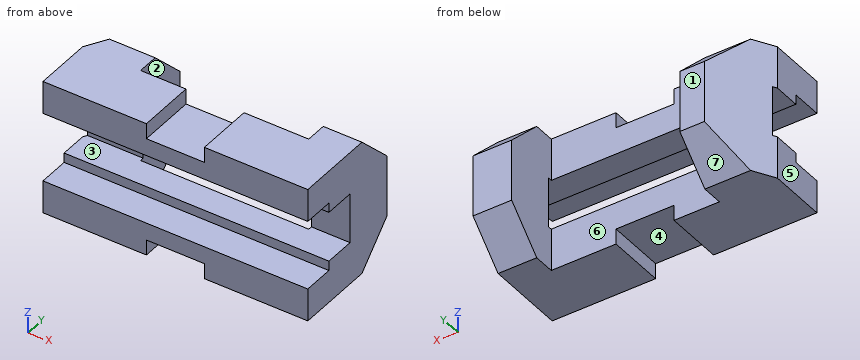
Autodesk Inventor part; units mm, degrees
ref_plane "YZ Plane" through (0, 0, 0) normal (1, 0, 0) x (0, 1, 0)
ref_plane "XZ Plane" through (0, 0, 0) normal (0, 1, 0) x (-1, 0, 0)
ref_plane "XY Plane" through (0, 0, 0) normal (0, 0, 1) x (1, 0, 0)
sketch "草圖1" plane through (0, 0, 0) normal (1, 0, 0) x (0, 1, 0)
  line L0 (-32, 35) -> (9, 35)
  line L1 (9, 35) -> (28, 16)
  line L2 (28, 16) -> (28, 0)
  line L3 (-32, 35) -> (-32, 18)
  line L4 (-32, 18) -> (-16, 18)
  line L5 (-16, 18) -> (-16, 13)
  line L6 (-16, 13) -> (0, 13)
  line L7 (0, 13) -> (0, 6.0328)
  line L8 (28, 0) -> (52.708, 0)
  line L9 (-32, -35) -> (9, -35)
  line L10 (9, -35) -> (28, -16)
  line L11 (28, -16) -> (28, 0)
  line L12 (-32, -35) -> (-32, -18)
  line L13 (-32, -18) -> (-16, -18)
  line L14 (-16, -18) -> (-16, -13)
  line L15 (-16, -13) -> (0, -13)
  line L16 (0, -13) -> (0, 6.0328)
  point P0 (0, 0)
  dimension "d0" = 19
  dimension "d1" = 70
  dimension "d2" = 26
  dimension "d3" = 36
  dimension "d4" = 32
  dimension "d5" = 60
  dimension "d6" = 16
  dimension "d7" = 0
  dimension "d8" = 19
extrude "擠出1" add sketch "草圖1" against normal blind 137
sketch "草圖2" plane through (0, -32, 35) normal (0, 0, 1) x (1, 0, 0)
  line L0 (-137, 0) -> (-137, 41)
  line L1 (-137, 30) -> (-119.6795, 60)
  line L2 (0, 60) -> (-137, 60)
  line L3 (-137, 60) -> (-137, 30)
  line L4 (-119.6795, 60) -> (-137, 60)
  point P0 (0, 32)
  dimension "d12" = 30
  dimension "d13" = 30
extrude "擠出2" cut sketch "草圖2" against normal blind 137
sketch "草圖3" plane through (0, -32, 35) normal (0, 0, 1) x (1, 0, 0)
  line L0 (0, 60) -> (-119.6795, 60)
  line L1 (-107, 60) -> (-20, 60)
  line L2 (-20, 60) -> (-20, 30)
  line L3 (-20, 30) -> (-107, 30)
  line L4 (-107, 30) -> (-107, 60)
  line L5 (-137, 0) -> (-137, 30)
  point P0 (0, 32)
  dimension "d16" = 30
  dimension "d17" = 30
  dimension "d18" = 87
extrude "擠出3" cut sketch "草圖3" against normal blind 137
sketch "草圖4" plane through (-107, -2, 35) normal (0, 1, 0) x (1, 0, 0)
  line L0 (87, 0) -> (0, 0)
  line L1 (23.5, 0) -> (53.5, 0)
  line L2 (53.5, 0) -> (53.5, 8)
  line L3 (53.5, 8) -> (23.5, 8)
  line L4 (23.5, 8) -> (23.5, 0)
  line L5 (107, 70) -> (-30, 70)
  line L6 (23.5, 70) -> (53.5, 70)
  line L7 (53.5, 70) -> (53.5, 62)
  line L8 (53.5, 62) -> (23.5, 62)
  line L9 (23.5, 62) -> (23.5, 70)
  line L10 (-30, 0) -> (-30, 22)
  line L11 (-30, 48) -> (-30, 70)
  point P0 (107, 35)
  dimension "d21" = 53.5
  dimension "d22" = 53.5
  dimension "d23" = 30
  dimension "d24" = 30
  dimension "d25" = 8
  dimension "d26" = 8
extrude "擠出4" cut sketch "草圖4" against normal blind 137
properties part number "410571040-2"
Can you work these out from the model? Positions are in its coordinate system, mm. Face numbers are marked on the shaded views. A direction names the side the tool comes from. Round coordinates to 2 decimals unless told otherwise and drop trailing zeros. Order: outer loops, then holes, each group sorted by start corner. A loop starts at its lowest first (then second) coordinate and runs counter-clockwise, first axis right, second up. Notation, with made-up numbers: (72.25, 53) -> (89.25, 53) arc R9 cw to (89.25, 66) -> close; hole circle Ø1 at (-34, 5.25). An arc over 180 degrees is marked (long way). Write each question's results on one line, items separated by ' | '. Start each with the question number.
Item 1: If we section it at C-C, the plane x = -72: Write out the boundary of the cut face in (y, z).
Item 2: Which directions (+Z, -Z, +X, -X, +Y, -Y) give clear straight access to the entire face, cutting with the end or side of a thin tool? Please do the marked faces 1, 2 and 3.
Item 3: If we section it at D-D, the plane x = -110: Write out the boundary of the cut face in (y, z).
Item 4: Will these pins go through, and if not, where does the flat tip stop? pin 1 (11 mm diameter, centred on x = -54.5, z = 26, fed in from +Y); pin 2 (6 mm diameter, centred on x = -14.5, z = 2.5, fed in from -Y); pin 3 (6 mm diameter, centred on y = 11, z = -28, fed in from -X).
Item 5: If we section it at A-A, the plane z = -1: Write out the boundary of the cut face in (x, y).
Item 6: Please list where these lines run through material, in increasing order: L1, parallel to Z at x = -17, y = -26; L2, parallel to Z at x = -49.5, y = -3; L3, parallel to X at y = 2.5, z = 8.5.
Item 7: If we section it at B-B, the plane y = -5.5: Write out the boundary of the cut face in (x, z).
Item 8: Thinking about a two-plate mould opening in X: for the marked faces 4, 5, 6 and 7, which applies, +X half, -X half, draft (parallel to the pull), parting line (faces both ways), or undercut?
Results:
1) outline: (-32, -27) -> (-2, -27) -> (-2, -13) -> (-16, -13) -> (-16, -18) -> (-32, -18) -> close; (-32, 18) -> (-16, 18) -> (-16, 13) -> (-2, 13) -> (-2, 27) -> (-32, 27) -> close
2) face 1: +Z, -Z, +X, -X, +Y | face 2: +Z, -Z, +Y | face 3: +X, -X, -Y
3) outline: (-32, -35) -> (9, -35) -> (28, -16) -> (28, 16) -> (9, 35) -> (-32, 35) -> (-32, 18) -> (-16, 18) -> (-16, 13) -> (0, 13) -> (0, -13) -> (-16, -13) -> (-16, -18) -> (-32, -18) -> close
4) pin 1: stops at y = -2 | pin 2: stops at y = 0 | pin 3: stops at x = -131.23
5) outline: (-135.85, 0) -> (-107, 0) -> (-107, 28) -> (-119.68, 28) -> close; (-20, 0) -> (0, 0) -> (0, 28) -> (-20, 28) -> close
6) L1: z = -35 to -18, 18 to 35 | L2: z = -35 to -13, 13 to 35 | L3: x = -134.4 to -107, -20 to 0
7) outline: (-137, -35) -> (-83.5, -35) -> (-83.5, -27) -> (-53.5, -27) -> (-53.5, -35) -> (0, -35) -> (0, -13) -> (-137, -13) -> close; (-137, 13) -> (0, 13) -> (0, 35) -> (-53.5, 35) -> (-53.5, 27) -> (-83.5, 27) -> (-83.5, 35) -> (-137, 35) -> close
8) face 4: undercut | face 5: -X half | face 6: undercut | face 7: draft
